Here's how the part is built. I have some questions about the finished solid (model axes, mm). A direction names the side the tool comes from. Give positions to 0.01 mm unless a question says otherwise; leave off trailing zeros. Write each loop counter-clockwise with the first axis right and the second up, starting at its lowest first coordinate (ties: lowest second). Pieces come first, ordered by that corner, then holes. Notation, with made-up numbers: (32.5, 67) -> (90.5, 67) arc R28 ccw to (90.5, 104) -> close; hole circle Ø9 at (62.25, 67). An arc over 180 degrees is marked (long way). Use CSV: the item, a comma, the result in double quotes. Start each with the question number.
(1) Which directions (+Z, -Z, +X, -X, +Y, -Y) give clear straight access to the entire face, cutting with the end or side of a thin tool? Please do faces 5 (the flat face through (-50, -2, -8)), 6 (the cylindrical face through (-47.586, -1.014, -8.753)).
(2) If we mould it in two halves opening along X, with no side actions, what happens to faces 1 (the cylindrical face through (-71.855, 4.437, -8.539)), 2 (the cylindrical face through (-65.516, 10.479, -8.753)), 3 (the cylindrical face through (-45.857, 4.437, -8.362)), 4 (the cylindrical face through (-56.57, 3.55, -8.51))? For each: pulls with the +X half, pulls with the -X half, needs draft (parallel to the pull), parting line crosses it, or undercut.
(3) Suppose I cut it at B-B on z = -8.25. List the corners of the cut face in (x, y) for me (3 decimals).
(4) Suppose I cut it at C-C on x = -60.25. List the corners of the cut face in (y, z) for me.
(5) Suppose I cut it at A-A on y = 4.5. List the corners of the cut face in (x, z) for me (3 decimals), plus the area to 3 significant figures.
(6) For pin 1 Ø2.5 at (x, z) = (-63.5, -7.5) entering from +Y; pin 2 Ø8 at (x, y) = (-57.5, 5) entering from +Z; pin 3 Ø2 at (y, z) = (3.5, -11) entering from -X; pin 4 Ø3 at (x, z) = (-63.5, -8.5) entering from -Y, each with a flat end and sliding along its axis, tell me the tip position at first contact or that it passes through.
(7) Suppose I cut it at D-D on x = -66.5. List the corners of the cut face in (y, z) for me.
(8) I need wall thicknesses on L1, parallel to Y at x = -65, z = -10.5; L2, parallel to X at y = 2.5, z = -12; L3, parallel to X at y = 0.5, z = -11.75. Which ranges of each line are inside material? Lowest first, please. Write a range as [from, to].
from build123d import *

# Parameters (mm, degrees)
BOSS_EXTRUDE2_DEPTH      = 9
CUT_EXTRUDE2_START       = -12.485338913
CUT_EXTRUDE2_OUTLINE_R   = 2.475
CUT_EXTRUDE2_DEPTH       = 8.07
BOSS_EXTRUDE3_DEPTH      = 9
BOSS_EXTRUDE3_DEPTH_BACK = 2
SKETCH1_6_R              = 2.325
SKETCH1_7_R              = 2.325
BOSS_EXTRUDE4_DEPTH      = 12


# Read off the part's stored shape, not the designer's step: Cut-Extrude2
with BuildPart() as part:
    # Sketch1 → Boss-Extrude2 (new body)
    with BuildSketch(Plane(origin=(0, 0, 0), x_dir=(1, 0, 0), z_dir=(0, 1, 0))):
        with BuildLine():
            Line((-49.891335879, 12.485338913), (-67.821335879, 12.485338913))
            ThreePointArc((-67.821335879, 12.485338913), (-71.856335879, 8.450338913), (-67.821335879, 4.415338913))
            Line((-67.821335879, 4.415338913), (-49.891335879, 4.415338913))
            ThreePointArc((-49.891335879, 4.415338913), (-45.856335879, 8.450338913), (-49.891335879, 12.485338913))
        make_face()
    extrude(amount=BOSS_EXTRUDE2_DEPTH)

    # Cut-Extrude2 outline → Cut-Extrude2 (cut)
    with BuildSketch(Plane.XY.offset(CUT_EXTRUDE2_START)):
        with Locations((-58.856335879, 4.5)):
            Circle(CUT_EXTRUDE2_OUTLINE_R)
    extrude(amount=CUT_EXTRUDE2_DEPTH, mode=Mode.SUBTRACT)

    # Sketch1<6> → Boss-Extrude3 (add, two sides: drawn at the far end of the back side and taken through both)
    with BuildSketch(Plane(origin=(0, 0, 0), x_dir=(1, 0, 0), z_dir=(0, 1, 0)).offset(-BOSS_EXTRUDE3_DEPTH_BACK)):
        with Locations(Location((-49.891335879, 8.450338913, 0), (0, 0, 270))):
            Circle(SKETCH1_6_R)
    extrude(amount=BOSS_EXTRUDE3_DEPTH + BOSS_EXTRUDE3_DEPTH_BACK)

    # Sketch1<7> → Boss-Extrude4 (add)
    with BuildSketch(Plane(origin=(0, 0, 0), x_dir=(1, 0, 0), z_dir=(0, 1, 0))):
        with Locations(Location((-67.821335879, 8.450338913, 0), (0, 0, 270))):
            Circle(SKETCH1_7_R)
    extrude(amount=BOSS_EXTRUDE4_DEPTH)


solid = part.part
Geometry says:
1,face 5,"+Z, -Z, +X, -X, -Y"
1,face 6,"-Y"
2,face 1,"pulls with the -X half"
2,face 2,"parting line crosses it"
2,face 3,"pulls with the +X half"
2,face 4,"undercut"
3,outline,"(-71.851, 0) -> (-52.208, 0) -> (-52.208, -2) -> (-47.575, -2) -> (-47.575, 0) -> (-45.861, 0) -> (-45.861, 9) -> (-65.505, 9) -> (-65.505, 12) -> (-70.138, 12) -> (-70.138, 9) -> (-71.851, 9) -> close; hole circle Ø4.95 at (-58.856, 4.5)"
4,outline,"(0, -12.49) -> (2.45, -12.49) -> (2.45, -4.42) -> (0, -4.42) -> close; (6.55, -12.49) -> (9, -12.49) -> (9, -4.42) -> (6.55, -4.42) -> close"
5,outline,"(-67.821, -12.485) -> (-61.331, -12.485) -> (-61.331, -4.415) -> (-67.821, -4.415) arc R4.035 ccw to start; (-56.381, -12.485) -> (-49.891, -12.485) arc R4.035 ccw to (-49.891, -4.415) -> (-56.381, -4.415) -> close"
5,area,"156 mm²"
6,pin 1,"y = 9"
6,pin 2,"z = -4.42"
6,pin 3,"x = -71.55"
6,pin 4,"y = 0"
7,outline,"(0, -12.49) -> (9, -12.49) -> (9, -10.36) -> (12, -10.36) -> (12, -6.54) -> (9, -6.54) -> (9, -4.42) -> (0, -4.42) -> close"
8,L1,"[0, 9]"
8,L2,"[-69.74, -60.31], [-57.4, -47.97]"
8,L3,"[-70.14, -47.57]"
